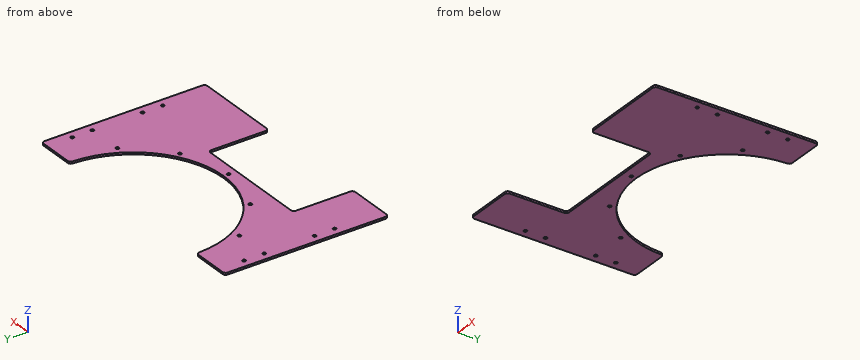
from build123d import *

# Parameters (mm, degrees)
SKETCH_1_W          = 260
SKETCH_1_H          = 163
EXTRUDE_1_DEPTH     = 2
SKETCH_2_R          = 1.6
CUT_EXTRUDE_1_DEPTH = 2
FILLET_1_R          = 3
SKETCH_3_R          = 90
SKETCH_3_R_2        = 1.6
CUT_EXTRUDE_2_DEPTH = 2
SKETCH_4_W          = 120
SKETCH_4_H          = 60
CUT_EXTRUDE_3_DEPTH = 2
FILLET_2_R          = 3


with BuildPart() as part:
    # 草图1 → 凸台-拉伸1 (new body)
    with BuildSketch(Plane.XY):
        Rectangle(SKETCH_1_W, SKETCH_1_H)
    extrude(amount=EXTRUDE_1_DEPTH)

    # 草图2 → 切除-拉伸1 (cut)
    with BuildSketch(Plane.XY.offset(2)):
        with Locations((-122, -33.5)):
            Circle(SKETCH_2_R)
        with Locations((-122, -13.5)):
            Circle(SKETCH_2_R)
        with Locations((-122, 36.5)):
            Circle(SKETCH_2_R)
        with Locations((-122, 56.5)):
            Circle(SKETCH_2_R)
        with Locations(Location((122, 56.5, 0), (0, 0, 180))):
            Circle(SKETCH_2_R)
        with Locations(Location((122, 36.5, 0), (0, 0, 180))):
            Circle(SKETCH_2_R)
        with Locations(Location((122, -13.5, 0), (0, 0, 180))):
            Circle(SKETCH_2_R)
        with Locations(Location((122, -33.5, 0), (0, 0, 180))):
            Circle(SKETCH_2_R)
    extrude(amount=-CUT_EXTRUDE_1_DEPTH, mode=Mode.SUBTRACT)

    # 圆角1
    fillet_1_edges = [part.edges().sort_by_distance(p)[0] for p in [
        (-130, 81.5, 1),
        (130, 81.5, 1),
        (130, -81.5, 1),
        (-130, -81.5, 1),
    ]]
    fillet(fillet_1_edges, radius=FILLET_1_R)

    # 草图3 → 切除-拉伸2 (cut)
    with BuildSketch(Plane.XY.offset(2)):
        with Locations((0, 81.5)):
            Circle(SKETCH_3_R)
        with Locations((0, -13.5)):
            Circle(SKETCH_3_R_2)
        with Locations((-50, -0.102540378)):
            Circle(SKETCH_3_R_2)
        with Locations((-86.602540378, 36.5)):
            Circle(SKETCH_3_R_2)
        with Locations((86.602540378, 36.5)):
            Circle(SKETCH_3_R_2)
        with Locations((50, -0.102540378)):
            Circle(SKETCH_3_R_2)
    extrude(amount=-CUT_EXTRUDE_2_DEPTH, mode=Mode.SUBTRACT)

    # 草图4 → 切除-拉伸3 (cut)
    with BuildSketch(Plane.XY.offset(2)):
        with Locations((-20, -51.5)):
            Rectangle(SKETCH_4_W, SKETCH_4_H)
    extrude(amount=-CUT_EXTRUDE_3_DEPTH, mode=Mode.SUBTRACT)

    # 圆角2
    fillet_2_edges = [part.edges().sort_by_distance(p)[0] for p in [
        (-80, -81.5, 1),
        (-80, -21.5, 1),
        (40, -21.5, 1),
        (40, -81.5, 1),
        (90, 81.5, 1),
        (-90, 81.5, 1),
    ]]
    fillet(fillet_2_edges, radius=FILLET_2_R)


solid = part.part
Work out the finished part from the listing and answer in its coordinate system (mm). Give positions to 0.01 mm unless a question says otherwise; leave off trailing zeros. Order: outer loops, then holes, each group sorted by start corner. A loop starts at its lowest first (then second) coordinate and runs counter-clockwise, first axis right, second up. Notation, with made-up numbers: M 2.25,3 L 56.25,3 A29 ccw 56.25,37 Z; hole C -27,-19.75 d6. An arc over 180 degrees is marked long. Return JSON: item names as keys, results as strings.
Q1. Find section A-A, the plane z = 1.65. State how many separate pieces and enclosed holes the cut face has, and give its area (3 significant figures).
Answer below:
{"separate pieces": "1", "enclosed holes": "13", "area": "22,300 mm^2"}
Q2. Find the intervals of material crossed by line 1 along Y through (x, z) = (122, 0.85); line 2 along X through (y, z) = (-61, 1.6); line 3 along X through (y, z) = (22.5, 0.25), in increasing order. Write a range as [from, to].
Answer below:
{"line 1": "y = [-81.5, -35.1], [-31.9, -15.1], [-11.9, 34.9], [38.1, 54.9], [58.1, 81.5]", "line 2": "x = [-130, -80], [40, 130]", "line 3": "x = [-130, -67.96], [67.96, 130]"}
Q3. Find section B-B, the plane x = -71. Write down the section's boundary in (y, z), and give its area (3 significant figures).
Answer below:
{"outline": "M -21.5,0 L 26.19,0 L 26.19,2 L -21.5,2 Z", "area": "95.4 mm^2"}
Q4. This flat-tipped pin is pushed along its axis until it touches: pin 1 (3.5 mm diameter, centred on x = 86.6, y = 36.5, fed in from +Z). Where does it stop, or does it pass through?
Answer below:
{"pin 1": "stops at z = 2"}
